Input: part model. Units: mm. Frame: model coordinates. Give positions to 0.01 mm unless a question says otherwise; leave off trailing zeros. Order: outer loops, then holes, each group sorted by start corner. A loop starts at its lowest first (then second) coordinate and runs counter-clockwise, first axis right, second up. Notation, with made-up numbers: (-23, 53.5) - (36, 53.5) arc R23 cw to (36, 72.5) - close; hole circle Ø2 at (68.25, -36). An arc over 180 degrees is marked (long way). Answer in a Markdown table with one row per item. Add a question column.
1. Section query B-B on x = -63.5. Return loops of the section in (y, z).
2. Section query C-C on z = 16.5. Return loops of the section in (x, y), and give its area (3 significant figures).
3. Section query A-A on y = -153. Return loops of the section in (x, z).
4. Ray query, line 1 (X direction, y = 118.5, z = 13); line 2 (X direction, y = -281.5, z = 22); line 3 (Y direction, x = -64, z = 9). Return the intervals inside material, ascending. Write a range as [from, to].
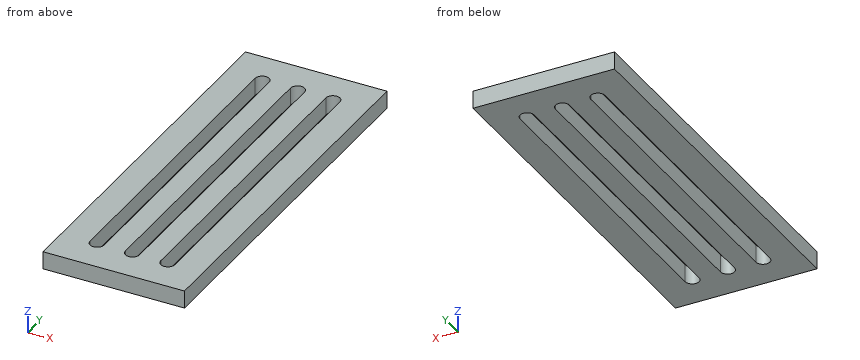
```python
from build123d import *

# Parameters (mm, degrees)
F0_W     = 254
F0_H     = 685.8
F1_DEPTH = 31.75


with BuildPart() as f1:
    # F0 (on Top) → F1 (new body)
    with BuildSketch(Plane.XY):
        Rectangle(F0_W, F0_H)
        with BuildLine():
            ThreePointArc((-76.2, 279.4), (-63.5, 292.1), (-50.8, 279.4))
            Line((-50.8, 279.4), (-50.8, -279.4))
            ThreePointArc((-50.8, -279.4), (-63.5, -292.1), (-76.2, -279.4))
            Line((-76.2, -279.4), (-76.2, 279.4))
        make_face(mode=Mode.SUBTRACT)
        with BuildLine():
            ThreePointArc((-12.7, 279.4), (0, 292.1), (12.7, 279.4))
            Line((12.7, 279.4), (12.7, -279.4))
            ThreePointArc((12.7, -279.4), (0, -292.1), (-12.7, -279.4))
            Line((-12.7, -279.4), (-12.7, 279.4))
        make_face(mode=Mode.SUBTRACT)
        with BuildLine():
            ThreePointArc((50.8, 279.4), (63.5, 292.1), (76.2, 279.4))
            Line((76.2, 279.4), (76.2, -279.4))
            ThreePointArc((76.2, -279.4), (63.5, -292.1), (50.8, -279.4))
            Line((50.8, -279.4), (50.8, 279.4))
        make_face(mode=Mode.SUBTRACT)
    extrude(amount=F1_DEPTH)


solid = f1.part
```
Answer:
| question | item | result |
|---|---|---|
| 1 | outline | (-342.9, 0) - (-292.1, 0) - (-292.1, 31.75) - (-342.9, 31.75) - close; (292.1, 0) - (342.9, 0) - (342.9, 31.75) - (292.1, 31.75) - close |
| 2 | outline | (-127, -342.9) - (127, -342.9) - (127, 342.9) - (-127, 342.9) - close; hole (-76.2, -279.4) arc R12.7 ccw to (-50.8, -279.4) - (-50.8, 279.4) arc R12.7 ccw to (-76.2, 279.4) - close; hole (-12.7, -279.4) arc R12.7 ccw to (12.7, -279.4) - (12.7, 279.4) arc R12.7 ccw to (-12.7, 279.4) - close; hole (50.8, -279.4) arc R12.7 ccw to (76.2, -279.4) - (76.2, 279.4) arc R12.7 ccw to (50.8, 279.4) - close |
| 2 | area | 130,000 mm² |
| 3 | outline | (-127, 0) - (-76.2, 0) - (-76.2, 31.75) - (-127, 31.75) - close; (-50.8, 0) - (-12.7, 0) - (-12.7, 31.75) - (-50.8, 31.75) - close; (12.7, 0) - (50.8, 0) - (50.8, 31.75) - (12.7, 31.75) - close; (76.2, 0) - (127, 0) - (127, 31.75) - (76.2, 31.75) - close |
| 4 | line 1 | x = [-127, -76.2], [-50.8, -12.7], [12.7, 50.8], [76.2, 127] |
| 4 | line 2 | x = [-127, -76.03], [-50.97, -12.53], [12.53, 50.97], [76.03, 127] |
| 4 | line 3 | y = [-342.9, -292.09], [292.09, 342.9] |
